```python
from build123d import *

# Parameters (mm, degrees)
SKETCH1_R           = 1.5
BOSS_EXTRUDE1_DEPTH = 7
FILLET1_R           = 5
FILLET2_R           = 3
SKETCH2_R           = 1.1
CUT_EXTRUDE1_DEPTH  = 28.212210096
CUT_EXTRUDE2_DEPTH  = 2.2
FILLET3_R           = 0.5


with BuildPart() as part:
    # Sketch1 → Boss-Extrude1 (new body)
    with BuildSketch(Plane(origin=(0, 0, 0), x_dir=(0, 0, -1), z_dir=(1, 0, 0))):
        with BuildLine():
            Line((0, -5), (-13.854054376, -10.750232807))
            Line((-13.854054376, -10.750232807), (-11.1706124, -17.215458183))
            Line((-11.1706124, -17.215458183), (9.071772057, -8.813699388))
            Line((9.071772057, -8.813699388), (4.618018125, 1.916744269))
            ThreePointArc((4.618018125, 1.916744269), (-4.158348311, 2.776353603), (0, -5))
        make_face()
        Circle(SKETCH1_R, mode=Mode.SUBTRACT)
    extrude(amount=BOSS_EXTRUDE1_DEPTH)

    # Fillet1
    fillet1_edges = [part.edges().sort_by_distance(p)[0] for p in [
        (3.5, -5, 0),
    ]]
    fillet(fillet1_edges, radius=FILLET1_R)

    # Fillet2
    fillet2_edges = [part.edges().sort_by_distance(p)[0] for p in [
        (7, -13.014578785, 1.049420171),
        (0, -9.423070941, 10.656519028),
        (7, -9.423070941, 10.656519028),
        (7, -3.44847756, -6.844895091),
        (0, -5.475900192, 4.79228393),
        (7, -5.475900192, 4.79228393),
        (7, 4.653790231, 1.828178461),
        (0, -3.44847756, -6.844895091),
        (0, -13.014578785, 1.049420171),
        (0, 4.653790231, 1.828178461),
    ]]
    fillet(fillet2_edges, radius=FILLET2_R)

    # Sketch2 → Cut-Extrude1 (cut, through all)
    with BuildSketch(Plane(origin=(0, -6.485014526, 15.624366332), x_dir=(1, 0, 0), z_dir=(0, -0.383348854, 0.923603625))):
        with Locations((3.5, -8.118018125)):
            Circle(SKETCH2_R)
    extrude(amount=-CUT_EXTRUDE1_DEPTH, mode=Mode.SUBTRACT)

    # Sketch3 → Cut-Extrude2 (cut)
    with BuildSketch(Plane.ZY):
        Polygon((2.385343934, 1.827610275), (-0.39008496, 2.979573581), (-2.775428893, 1.151963306), (-2.385343934, -1.827610275), (0.39008496, -2.979573581), (2.775428893, -1.151963306), align=None)
    extrude(amount=-CUT_EXTRUDE2_DEPTH, mode=Mode.SUBTRACT)

    # Fillet3
    fillet3_edges = [part.edges().sort_by_distance(p)[0] for p in [
        (0, -13.982845495, 12.512333388),
        (7, -13.982845495, 12.512333388),
        (3.5, -10.750232807, 13.854054376),
        (3.5, -17.215458183, 11.1706124),
        (6.121320344, -16.403906467, 11.507453239),
        (6.121320344, -11.561784523, 13.517213537),
        (0.878679656, -16.403906467, 11.507453239),
        (0.878679656, -11.561784523, 13.517213537),
    ]]
    fillet(fillet3_edges, radius=FILLET3_R)


solid = part.part
```
The listing builds one solid part. Answer for the finished solid, in the listing's coordinates (mm). A direction names the side the tool comes from. Coordinates: 2 decimals unless noted, no trailing zeros. Loops run counter-clockwise (first coordinate to the right, second up) from the corner with the lowest first, then second, coordinate; pieces in that order, holes last. Notation, with made-up numbers: M 78.5,-31.5 L 131.5,-31.5 A20 cw 131.5,6.5 Z; hole C 63.5,88.25 d3. An arc over 180 degrees is marked long. Answer as CSV lines item,"result". Start each with the question number.
(1) The part is cut by section B-B (z = 0). State how many separate pieces and enclosed holes the cut face has, and give its area (3 significant figures).
(2) Find the intervals of material crossed by L1, parallel to Y at x = 3.55, z = 0; L2, parallel to Z at x = 6.5, y = -1; L3, parallel to Z at x = 5.55, y = 0, in increasing order. Write a range as [from, to].
(3) Given pin 1 (3 mm diameter, centred on y = -9, z = 9.5, fed in from -X); pin 2 (3 mm diameter, centred on x = 2.5, y = 2.5, fed in from -Z); pin 3 (2.5 mm diameter, centred on y = 0, z = 0, fed in from -X); pin 4 (1.7 mm diameter, centred on y = 0.5, z = 0.5, fed in from -X), each flat-ended and moving along its own axis, determine where each tip first touches the part or whether it passes through.
(4) For faces 1 (the cylindrical face through (6.85, -13.922, 12.383)), 2 (the flat face through (1.116, 0.317, 2.583)), determine the directions among +Z, -Z, +X, -X, +Y, -Y from which every point of the face is accessible in a straight line to the end or side of a thin tool.
(5) The part is cut by section A-A (x = 3.5). Give the vertices of the cut face in (y, z), and give its area (3 significant figures).
(6) The mould has two halves that part along Y. Classify faces 3 (the flat face through (1.116, 2.079, -1.566)), 4 (the cylindrical face through (6.1, -3.7, -6.02)), 5 (the cylindrical face through (6.145, -12.028, 1.026)): pulls with the +Y half, pulls with the -Y half, needs draft (parallel to the pull), parting line crosses it, or undercut.
Determined:
1,separate pieces,"2"
1,enclosed holes,"1"
1,area,"84.1 mm2"
2,L1,"[-12.58, -9.98], [-7.6, -1.5], [1.5, 5]"
2,L2,"[-4.38, -1.12], [1.12, 3.52]"
2,L3,"[-4.95, -1.5], [1.5, 4.57]"
3,pin 1,"x = 0.37"
3,pin 2,"z = -4.98"
3,pin 3,"through"
3,pin 4,"x = 2.2"
4,face 1,"+Z, +X, -Y"
4,face 2,"-X"
5,outline,"M -17.02,10.71 L -8.81,-9.07 L -6.6,-8.15 L -15,12.09 L -16.75,11.36 A0.5 ccw Z; M -12.97,12.93 L -4.57,-7.31 L 1.92,-4.62 A5 ccw -1.74,4.69 A5 cw -8.1,7.46 L -10.56,13.39 A0.5 ccw -11.21,13.66 Z; hole C 0,0 d3"
5,area,"189 mm2"
6,face 3,"undercut"
6,face 4,"pulls with the +Y half"
6,face 5,"pulls with the -Y half"
